from build123d import *

# Parameters (mm, degrees)
BOSS_EXTRUDE1_START      = 20
SKETCH2_R                = 75.89
BOSS_EXTRUDE1_DEPTH      = 20
M3_CLEARANCE_HOLE1_D     = 3.24
M3_CLEARANCE_HOLE1_DEPTH = 156.298383092
M3_CLEARANCE_HOLE2_D     = 3.24
M3_CLEARANCE_HOLE2_DEPTH = 156.298383092
M3_CLEARANCE_HOLE3_D     = 3.24
M3_CLEARANCE_HOLE3_DEPTH = 156.298383092
HOLE1_REACH              = 178.309
HOLE1_BORE_R             = 2.46
M3_CLEARANCE_HOLE4_D     = 3.24
M3_CLEARANCE_HOLE4_DEPTH = 154.24
M3_CLEARANCE_HOLE5_D     = 3.24
M3_CLEARANCE_HOLE5_DEPTH = 154.798004693
M3_CLEARANCE_HOLE6_D     = 3.24
M3_CLEARANCE_HOLE6_DEPTH = 154.798004693
CHAMFER1_SIZE            = 0.25
CHAMFER2_SIZE            = 3


with BuildPart() as part:
    # Sketch1 → Revolve1 (revolve)
    with BuildSketch(Plane(origin=(0, 0, 0), x_dir=(-1, 0, 0), z_dir=(0, 0, -1)), mode=Mode.PRIVATE) as revolve1_sk:
        Polygon((-78.35, 0), (0, 0), (0, 24), (-75.89, 24), (-75.89, 22), (-73.64, 22), (-73.64, 18.4), (-75.89, 18.4), (-75.89, 4), (-78.35, 4), align=None)
    revolve(revolve1_sk.sketch.rotate(Axis((0, 0, 0), (0, 1, 0)), 270), axis=Axis((0, 0, 0), (0, 1, 0)))

    # Sketch2 → Boss-Extrude1 (add)
    with BuildSketch(Plane.XZ.offset(BOSS_EXTRUDE1_START)):
        with Locations(Location((0, 0, 0), (0, 0, 90))):
            Circle(SKETCH2_R)
    extrude(amount=-BOSS_EXTRUDE1_DEPTH)

    # Sketch3 → Cut-Revolve1 (revolve, cut)
    with BuildSketch(Plane.XY, mode=Mode.PRIVATE) as cut_revolve1_sk:
        Polygon((71.39, 24), (0, 24), (0, -20), (72.89, -20), (72.89, 0), (4.25, 0), (4.25, 4), (71.39, 4), align=None)
    revolve(cut_revolve1_sk.sketch.rotate(Axis((0, 24, 0), (0, -1, 0)), 270), axis=Axis((0, 24, 0), (0, -1, 0)), mode=Mode.SUBTRACT)

    # M3 Clearance Hole1
    with Locations(Plane(origin=(65.722667893, 14, -37.945), x_dir=(0.5, 0, 0.866025403784), z_dir=(0.866025403784, 0, -0.5))):
        with Locations((0, 0)):
            Hole(M3_CLEARANCE_HOLE1_D / 2, depth=M3_CLEARANCE_HOLE1_DEPTH)

    # M3 Clearance Hole2
    with Locations(Plane(origin=(65.722667893, 14, 37.945), x_dir=(-0.5, 0, 0.866025403784), z_dir=(0.866025403784, 0, 0.5))):
        with Locations((0, 0)):
            Hole(M3_CLEARANCE_HOLE2_D / 2, depth=M3_CLEARANCE_HOLE2_DEPTH)

    # M3 Clearance Hole3
    with Locations(Plane(origin=(0, 14, 75.89), x_dir=(1, 0, 0), z_dir=(0, 0, 1))):
        with Locations((0, 0)):
            Hole(M3_CLEARANCE_HOLE3_D / 2, depth=M3_CLEARANCE_HOLE3_DEPTH)

    # Hole1 bore (on position points) → Hole1 (cut, up to next)
    with BuildSketch(Plane(origin=(75.89, -10, 0), x_dir=(0, 0, 1), z_dir=(1, 0, 0)), mode=Mode.PRIVATE) as hole1_sk1:
        Circle(HOLE1_BORE_R)
    hole1_tool1 = extrude(hole1_sk1.sketch, amount=-HOLE1_REACH, mode=Mode.PRIVATE) & part.part
    add(hole1_tool1.solids().sort_by_distance((75.89, -10, 0))[0], mode=Mode.SUBTRACT)

    # M3 Clearance Hole4
    with Locations(Plane(origin=(-75.89, -10, 0), x_dir=(0, 0, -1), z_dir=(-1, 0, 0))):
        with Locations((0, 0)):
            Hole(M3_CLEARANCE_HOLE4_D / 2, depth=M3_CLEARANCE_HOLE4_DEPTH)

    # M3 Clearance Hole5
    with Locations(Plane(origin=(37.945, -10, -65.722667893), x_dir=(-0.866025403784, 0, -0.5), z_dir=(0.5, 0, -0.866025403784))):
        with Locations((0, 0)):
            Hole(M3_CLEARANCE_HOLE5_D / 2, depth=M3_CLEARANCE_HOLE5_DEPTH)

    # M3 Clearance Hole6
    with Locations(Plane(origin=(37.945, -10, 65.722667893), x_dir=(0.866025403784, 0, -0.5), z_dir=(0.5, 0, 0.866025403784))):
        with Locations((0, 0)):
            Hole(M3_CLEARANCE_HOLE6_D / 2, depth=M3_CLEARANCE_HOLE6_DEPTH)

    # Chamfer1
    chamfer1_edges = [part.edges().sort_by_distance(p)[0] for p in [
        (0, 24, -75.89),
        (0, 0, -78.35),
        (0, -20, -75.89),
        (0, 24, 71.39),
        (0, -20, 72.89),
        (0, 4, -78.35),
    ]]
    chamfer(chamfer1_edges, length=CHAMFER1_SIZE)

    # Chamfer2
    chamfer2_edges = [part.edges().sort_by_distance(p)[0] for p in [
        (0, 0, 72.89),
        (0, 4, 71.39),
    ]]
    chamfer(chamfer2_edges, length=CHAMFER2_SIZE)


solid = part.part
The listing builds one solid part. Answer for the finished solid, in the listing's coordinates (mm). A direction names the side the tool comes from. Give positions to 0.01 mm unless a question says otherwise; leave off trailing zeros. Answer as a JSON object with one key per item and string values.
1. For faces 4 (the flat face through (-15, 0, 1)), 5 (the cylindrical face through (22.795, 11.099, 72.386)), 6 (the cylindrical face through (74.39, -7.598, -0.533)), determine the directions among +Z, -Z, +X, -X, +Y, -Y from which every point of the face is accessible in a straight line to the end or side of a thin tool.
Determined:
{"face 4": "-Y", "face 5": "+Y", "face 6": "+X"}
2. For a pull along Z with two mould halves and no side action, classify faces 1 (the flat face through (76, 4, 12)), 2 (the cylindrical face through (-44.352, -11.258, 57.843)), 3 (the cylindrical face through (22.795, 22.863, 72.386)) as pulls with the +Z half, pulls with the -Z half, needs draft (parallel to the pull), parting line crosses it, or undercut.
Determined:
{"face 1": "needs draft", "face 2": "undercut", "face 3": "parting line crosses it"}
3. Flat-ended cylindrical pins translate along their axes: pin 1 Ø6 at (x, y) = (-0.5, -5) entering from +Z; pin 2 Ø2 at (x, y) = (-34.5, 10) entering from +Z; pin 3 Ø1.9 at (x, y) = (0, 14) entering from -Z; pin 4 Ø13.5 at (x, z) = (0, 0) entering from -Y. Find the tip coordinate at first contact, or state that the pin passes through.
Determined:
{"pin 1": "z = 75.89", "pin 2": "z = 68.1", "pin 3": "through", "pin 4": "y = 0"}
4. Find the intervals of material crossed by L1, parallel to Y at x = -74.7, z = 0; L2, parallel to X at y = -7.75, z = 0; L3, parallel to Y at x = 26, z = 12, in increasing order. Write a range as [from, to].
Determined:
{"L1": "[-20, -11.62], [-8.38, 18.4], [22, 24]", "L2": "[-75.89, -72.89]", "L3": "[0, 4]"}
